Read the model definition and answer for the solid it produces. Units are mm, in the model's axes. A direction names the side the tool comes from. Round coordinates to 2 decimals unless told otherwise and drop trailing zeros. Order: outer loops, then holes, each group sorted by start corner. A loop starts at its lowest first (then second) coordinate and runs counter-clockwise, first axis right, second up.
from build123d import *

# Parameters (mm, degrees)
BOSS_EXTRUDE1_DEPTH = 11
SKETCH3_W           = 22
SKETCH3_H           = 3
BOSS_EXTRUDE2_DEPTH = 17.7
BOSS_EXTRUDE3_DEPTH = 5
SKETCH5_R           = 1.75
CUT_EXTRUDE1_DEPTH  = 37.035744466
SKETCH6_W           = 9
SKETCH6_H           = 9
BOSS_EXTRUDE4_DEPTH = 5
SKETCH7_R           = 2.25
CUT_EXTRUDE2_DEPTH  = 38.573063213
FILLET1_R           = 1
SKETCH8_R           = 2.5
CUT_EXTRUDE3_DEPTH  = 0.75
FILLET2_R           = 0.5


with BuildPart() as part:
    # Sketch1 → Boss-Extrude1 (new, symmetric)
    with BuildSketch(Plane(origin=(0, 0, 0), x_dir=(0, 0, -1), z_dir=(1, 0, 0))):
        Polygon((-13.0089, 0), (13.0089, 0), (13.0089, 10.5), (5.7589, 10.5), (5.7589, 9), (-5.7589, 9), (-5.7589, 10.5), (-13.0089, 10.5), align=None)
    extrude(amount=BOSS_EXTRUDE1_DEPTH, both=True)

    # Sketch3 → Boss-Extrude2 (add)
    with BuildSketch(Plane.XZ):
        with Locations((0, -14.5089)):
            Rectangle(SKETCH3_W, SKETCH3_H)
        with Locations((0, 14.5089)):
            Rectangle(SKETCH3_W, SKETCH3_H)
    extrude(amount=-BOSS_EXTRUDE2_DEPTH)

    # Sketch4 → Boss-Extrude3 (add)
    with BuildSketch(Plane(origin=(11, 0, 0), x_dir=(0, 0, -1), z_dir=(1, 0, 0))):
        Polygon((-8.8, 17.7), (-16.0089, 17.7), (-16.0089, 0), (16.0089, 0), (16.0089, 17.7), align=None)
    extrude(amount=BOSS_EXTRUDE3_DEPTH)

    # Sketch5 → Cut-Extrude1 (cut, through all)
    with BuildSketch(Plane(origin=(16, 0, 0), x_dir=(0, 0, -1), z_dir=(1, 0, 0))):
        with Locations((-10.5, 13)):
            Circle(SKETCH5_R)
        with Locations((10.5, 13)):
            Circle(SKETCH5_R)
    extrude(amount=-CUT_EXTRUDE1_DEPTH, mode=Mode.SUBTRACT)

    # Sketch6 → Boss-Extrude4 (add)
    with BuildSketch(Plane.XZ):
        with Locations((20.5, 0)):
            Rectangle(SKETCH6_W, SKETCH6_H)
        with Locations((2.5, 20.5089)):
            Rectangle(SKETCH6_W, SKETCH6_H)
    extrude(amount=-BOSS_EXTRUDE4_DEPTH)

    # Sketch7 → Cut-Extrude2 (cut, through all)
    with BuildSketch(Plane(origin=(0, 5, 0), x_dir=(1, 0, 0), z_dir=(0, 1, 0))):
        with Locations(Location((20.5, 0, 0), (0, 0, 270))):
            Circle(SKETCH7_R)
        with Locations(Location((2.5, -20.5089, 0), (0, 0, 270))):
            Circle(SKETCH7_R)
    extrude(amount=-CUT_EXTRUDE2_DEPTH, mode=Mode.SUBTRACT)

    # Fillet1
    fillet1_edges = [part.edges().sort_by_distance(p)[0] for p in [
        (0, 10.5, 5.7589),
        (0, 10.5, -5.7589),
        (0, 17.7, -13.0089),
        (11, 14.1, -13.0089),
        (11, 14.1, 13.0089),
        (0, 17.7, 13.0089),
        (11, 17.7, 0),
        (25, 5, 0),
        (25, 2.5, 4.5),
        (25, 2.5, -4.5),
        (7, 2.5, 25.0089),
        (2.5, 5, 25.0089),
        (-2, 2.5, 25.0089),
    ]]
    fillet(fillet1_edges, radius=FILLET1_R)

    # Sketch8 → Cut-Extrude3 (cut)
    with BuildSketch(Plane(origin=(16, 0, 0), x_dir=(0, 0, -1), z_dir=(1, 0, 0))):
        with Locations((-10.5, 13)):
            Circle(SKETCH8_R)
        with Locations((10.5, 13)):
            Circle(SKETCH8_R)
    extrude(amount=-CUT_EXTRUDE3_DEPTH, mode=Mode.SUBTRACT)

    # Fillet2
    fillet2_edges = [part.edges().sort_by_distance(p)[0] for p in [
        (16, 13, 13),
        (16, 13, -8),
    ]]
    fillet(fillet2_edges, radius=FILLET2_R)


solid = part.part
Q1. A cutting plane is placed at A-A, the plane z = -10.5. Give the vertices of the cut face in (x, y).
Outcome:
outline: (-11, 0) - (16, 0) - (16, 10) arc R0.5 ccw to (15.5, 10.5) - (15.25, 10.5) - (15.25, 11.25) - (11, 11.25) - (11, 10.5) - (-11, 10.5) - close; (11, 14.75) - (15.25, 14.75) - (15.25, 15.5) - (15.5, 15.5) arc R0.5 ccw to (16, 16) - (16, 17.7) - (12, 17.7) arc R1 ccw to (11, 16.7) - close
Q2. A cutting plane is placed at D-D, the plane z = 0. Give the vertices of the cut face in (x, y).
Outcome:
outline: (-11, 0) - (18.25, 0) - (18.25, 5) - (16, 5) - (16, 17.7) - (12, 17.7) arc R1 ccw to (11, 16.7) - (11, 9) - (-11, 9) - close; (22.75, 0) - (25, 0) - (25, 4) arc R1 ccw to (24, 5) - (22.75, 5) - close
Q3. For faces 5 (the face through (3, 5, 18)), 6 (the face through (11.301, 17.415, 0.168)), 7 (the face through (18, 5, 0)), determine the directions among +Z, -Z, +X, -X, +Y, -Y from which every point of the face is accessible in a straight line to the end or side of a thin tool.
Outcome:
face 5: +Z, +X, -X, +Y
face 6: -X, +Y
face 7: +Z, -Z, +X, +Y
Q4. A cutting plane is placed at C-C, the plane y = 2.25. Give the vertices of the cut face in (x, z).
Outcome:
outline: (-11, -16.01) - (16, -16.01) - (16, -4.5) - (24, -4.5) arc R1 ccw to (25, -3.5) - (25, 3.5) arc R1 ccw to (24, 4.5) - (16, 4.5) - (16, 16.01) - (7, 16.01) - (7, 24.01) arc R1 ccw to (6, 25.01) - (-1, 25.01) arc R1 ccw to (-2, 24.01) - (-2, 16.01) - (-11, 16.01) - close; hole circle Ø4.5 at (2.5, 20.51); hole circle Ø4.5 at (20.5, 0)
Q5. A cutting plane is placed at B-B, the plane x = 2.5. Give the vertices of the cut face in (y, z), plus the area to 3 significant figures.
Outcome:
outline: (0, -16.01) - (17.7, -16.01) - (17.7, -14.01) arc R1 ccw to (16.7, -13.01) - (10.5, -13.01) - (10.5, -6.76) arc R1 ccw to (9.5, -5.76) - (9, -5.76) - (9, 5.76) - (9.5, 5.76) arc R1 ccw to (10.5, 6.76) - (10.5, 13.01) - (16.7, 13.01) arc R1 ccw to (17.7, 14.01) - (17.7, 16.01) - (5, 16.01) - (5, 18.26) - (0, 18.26) - close; (0, 22.76) - (5, 22.76) - (5, 24.01) arc R1 ccw to (4, 25.01) - (0, 25.01) - close
area: 384 mm2
Q6. For a pull along Z with two mould halves and no side action, classify faces 1 (the face through (13.155, 14.735, -10.272)), 2 (the face through (2.563, 4.715, 24.708)), 3 (the face through (2, 9, -16.009)), 4 (the face through (10.715, 15.313, -12.708)) as released by +Z, released by -Z, zero draft, split by the parting line, or undercut.
Outcome:
face 1: undercut
face 2: released by +Z
face 3: released by -Z
face 4: undercut
Q7. Straight lines are drawn through the part: probe 1 along Z at (x, y) = (12.4, 13); probe 2 along X at (y, z) = (3.3, 0); probe 3 along Z at (x, y) = (-7, 9.5). For each, find the intervals that lie inside material, in ascending order.
Outcome:
probe 1: z = -16.01 to -12.25, -8.75 to 8.75, 12.25 to 16.01
probe 2: x = -11 to 18.25, 22.75 to 25
probe 3: z = -16.01 to -5.76, 5.76 to 16.01
Q8. Flat-ended cylindrical pins translate along their axes: pin 1 (9 mm diameter, centred on x = -4, y = 12.5, fed in from +Z); pin 2 (5 mm diameter, centred on x = 4.5, z = -9.5, fed in from +Y); pin 3 (2 mm diameter, centred on y = 4.5, z = 19.5, fed in from -X). Find the tip coordinate at first contact, or state that the pin passes through.
Outcome:
pin 1: stops at z = 16.01
pin 2: stops at y = 10.5
pin 3: stops at x = -2
